from build123d import *

# Parameters (mm, degrees)
BOSS_EXTRUDE1_DEPTH = 12.7
SKETCH2_R           = 1.905
CUT_EXTRUDE1_DEPTH  = 12.7


with BuildPart() as part:
    # Sketch1 → Boss-Extrude1 (new body)
    with BuildSketch(Plane.XY):
        with BuildLine():
            Line((0, 0), (0, 3.175))
            Line((0, 3.175), (-13.110280444, 3.175))
            Line((-13.110280444, 3.175), (-13.110280444, 9.525))
            Line((-13.110280444, 9.525), (-13.97, 9.525))
            Line((-13.97, 9.525), (-13.97, 10.795))
            Line((-13.97, 10.795), (-13.110280444, 10.795))
            Line((-13.110280444, 10.795), (-14.697780444, 13.544630657))
            Line((-14.697780444, 13.544630657), (-15.5575, 13.544630657))
            Line((-15.5575, 13.544630657), (-15.5575, 10.524942302))
            add(Edge.make_bspline(
                [(-14.697780444, 5.304098901), (-14.697780444, 8.859756712), (-15.501871983, 8.436070985), (-15.5575, 10.524942302)],
                knots=[0, 0, 0, 0, 1, 1, 1, 1], degree=3))
            Line((-14.697780444, 5.304098901), (-14.697780444, 0))
            Line((-14.697780444, 0), (0, 0))
        make_face()
    boss_extrude1 = extrude(amount=BOSS_EXTRUDE1_DEPTH)

    # Mirror1: Boss-Extrude1 across plane
    add(boss_extrude1.mirror(Plane(origin=(0, 0, 0), x_dir=(0, 0, 1), z_dir=(1, 0, 0))))

    # Sketch2 → Cut-Extrude1 (cut)
    with BuildSketch(Plane(origin=(0, 3.175, 0), x_dir=(1, 0, 0), z_dir=(0, 1, 0))):
        with Locations(Location((0, -6.35, 0), (0, 0, 270))):
            Circle(SKETCH2_R)
    extrude(amount=-CUT_EXTRUDE1_DEPTH, mode=Mode.SUBTRACT)


solid = part.part
Geometry check sheet. Reference: the model listing, model coordinates, mm. A direction names the side the tool comes from. Round coordinates to 2 decimals unless told otherwise and drop trailing zeros. Order: outer loops, then holes, each group sorted by start corner. A loop starts at its lowest first (then second) coordinate and runs counter-clockwise, first axis right, second up. Notation, with made-up numbers: (76, 50) -> (83, 50) arc R23 ccw to (83, 69) -> close; hole circle Ø6 at (5.25, 10.25). An arc over 180 degrees is marked (long way). Use one line per item in the form item = value.
1. Cross-section at A-A, the plane x = 0. Enter the section's corners in (y, z) (3 decimals), plus the area to 3 significant figures.
Working result:
outline = (0, 0) -> (3.175, 0) -> (3.175, 4.445) -> (0, 4.445) -> close; (0, 8.255) -> (3.175, 8.255) -> (3.175, 12.7) -> (0, 12.7) -> close
area = 28.2 mm^2
2. Mould release check, pull along Y, two halves, no side actions. Record for faces 1 (the face through (-15.558, 12, 6)), 2 (the face through (13.893, 12.151, 6.261)), 3 (the face through (13.97, 10, 6)): pulls with the +Y half, pulls with the -Y half, needs draft (parallel to the pull), parting line crosses it, or undercut.
Working result:
face_1 = needs draft
face_2 = pulls with the +Y half
face_3 = undercut
3. Scan lines: line 1 along X through (y, z) = (2.1, 6.35) (3 decimals); line 2 along Y through (x, z) = (-7, 7.25) (3 decimals); line 3 along Z through (x, y) = (1.5, 1.5). Record each from-to range of solid material in increasing order. Write a range as from..to.
Working result:
line_1 = -14.698..-1.905, 1.905..14.698
line_2 = 0..3.175
line_3 = 0..5.18, 7.52..12.7
4. Set-up check for faces 4 (the face through (-14.698, 3, 6)), 5 (the face through (14.698, 3, 6)), 6 (the face through (13.11, 6, 6)), 7 (the face through (13.5, 9.525, 6.3)): record each of +Z, -Z, +X, -X, +Y, -Y from which the full face is reachable in a straight line by a thin tool's end or side.
Working result:
face_4 = +Z, -Z, -X, -Y
face_5 = +Z, -Z, +X, -Y
face_6 = +Z, -Z, +Y
face_7 = +Z, -Z
5. Cross-section at B-B, the plane y = 4.5. Enter the section's corners in (x, z).
Working result:
outline = (-14.7, 0) -> (-13.11, 0) -> (-13.11, 12.7) -> (-14.7, 12.7) -> close; (13.11, 0) -> (14.7, 0) -> (14.7, 12.7) -> (13.11, 12.7) -> close
6. Cross-section at C-C, the plane x = 7.5. Enter the section's corners in (y, z) (3 decimals), plus the area to 3 significant figures.
Working result:
outline = (0, 0) -> (3.175, 0) -> (3.175, 12.7) -> (0, 12.7) -> close
area = 40.3 mm^2
7. Go/stop test with flat-tipped pins: pin 1 (1.6 mm diameter, centred on y = 1.5, z = 8.5, fed in from -X); pin 2 (1.9 mm diameter, centred on y = 7, z = 7, fed in from -X); pin 3 (6 mm diameter, centred on y = 2, z = 8, fed in from +X). Record where each tip stops, or that it passes through.
Working result:
pin_1 = -14.7
pin_2 = -14.95
pin_3 = 14.7
